Can you work these out from the model? Positions are in its coordinate system, mm. Face numbers are marked on the shaded views. A direction names the side the tool comes from. Give positions to 0.01 mm unless a question says otherwise; leave off trailing zeros. Write each loop counter-clockwise with the first axis right and the second up, starting at its lowest first coordinate (ties: lowest second). Pieces come first, ordered by that corner, then holes.
```python
from build123d import *

# Parameters (mm, degrees)
BOSS_EXTRUDE1_START = -9
BOSS_EXTRUDE1_DEPTH = 82
CHAMFER1_SIZE       = 0.5


with BuildPart() as part:
    # Sketch1 → Boss-Extrude1 (new body)
    with BuildSketch(Plane(origin=(0, 0, 0), x_dir=(0, 0, -1), z_dir=(1, 0, 0)).offset(BOSS_EXTRUDE1_START)):
        Polygon((0, 7.505553499), (-6.5, 3.75277675), (-6.5, -3.75277675), (0, -7.505553499), (6.5, -3.75277675), (6.5, 3.75277675), align=None)
    extrude(amount=BOSS_EXTRUDE1_DEPTH)

    # Sketch2 → Cut-Revolve1 (revolve, cut)
    with BuildSketch(Plane.XY, mode=Mode.PRIVATE) as cut_revolve1_sk:
        Polygon((0, 7.505553499), (-9, 7.505553499), (-9, 4), (-1, 4), (-1, 3.45), (0, 3.45), align=None)
    revolve(cut_revolve1_sk.sketch.rotate(Axis((-20.13204944, 0, 0), (1, 0, 0)), 90), axis=Axis((-20.13204944, 0, 0), (1, 0, 0)), mode=Mode.SUBTRACT)

    # Sketch3 → Cut-Revolve2 (revolve, cut)
    with BuildSketch(Plane.XY, mode=Mode.PRIVATE) as cut_revolve2_sk:
        Polygon((34.8, 7.505553499), (34.8, 4), (35.8, 4), (35.8, 3), (65, 3), (65, 2.5), (73, 2.5), (73, 7.505553499), align=None)
    revolve(cut_revolve2_sk.sketch.rotate(Axis((-14.24617289, 0, 0), (1, 0, 0)), 90), axis=Axis((-14.24617289, 0, 0), (1, 0, 0)), mode=Mode.SUBTRACT)

    # Sketch4 → Cut-Revolve3 (revolve, cut)
    with BuildSketch(Plane.XY, mode=Mode.PRIVATE) as cut_revolve3_sk:
        Polygon((34.8, 7.505553499), (34.075105849, 7.505553499), (34.8, 6.25), align=None)
    revolve(cut_revolve3_sk.sketch.rotate(Axis((-12.936203068, 0, 0), (1, 0, 0)), 90), axis=Axis((-12.936203068, 0, 0), (1, 0, 0)), mode=Mode.SUBTRACT)

    # Chamfer1
    chamfer1_edges = [part.edges().sort_by_distance(p)[0] for p in [
        (-9, 0, -4),
        (73, 0, -2.5),
    ]]
    chamfer(chamfer1_edges, length=CHAMFER1_SIZE)


solid = part.part
```
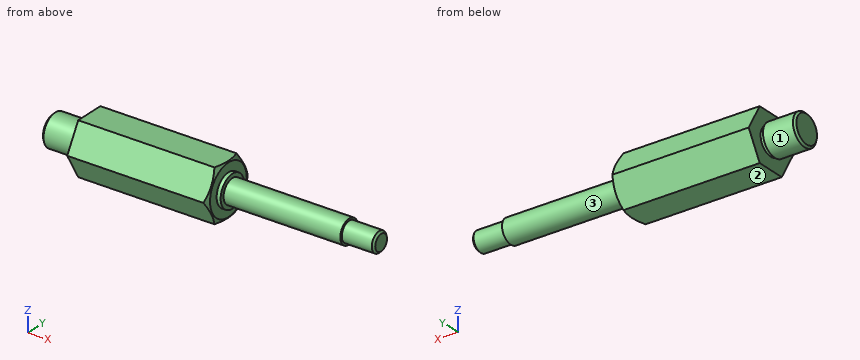
1) Please list where these lines run through material, in increasing order: L1, parallel to X at y = -3.75, z = 4.25; L2, parallel to X at y = 0.5, z = -2.75; L3, parallel to X at y = -0.75, z = 3.75.
Values follow:
L1: x = 0 to 34.8
L2: x = -9 to 65
L3: x = -8.68 to -1, 0 to 35.8
2) For the marked faces 1, 2 and 3, which set-ups out of +Z, -Z, +X, -X, +Y, -Y let a thin tool reach every point of the face, with its end or its side?
Values follow:
face 1: -X
face 2: -Z, +X, -X, +Y, -Y
face 3: +X
3) Suppose I cut it at C-C on x = 67. Write out the boundary of the cut face in (y, z), plus the area to 3 significant figures.
Values follow:
outline: circle Ø5 at (0, 0)
area: 19.6 mm2
4) For pin 1 Ø6 at (y, z) = (3, 1) entering from +X; pin 2 Ø8 at (x, y) = (62, 5.5) entering from +Z; pin 3 Ø4 at (x, y) = (64, -2.5) entering from +Z; pin 4 Ø6 at (x, y) = (60, 3.5) entering from -Z, each with a flat end and sliding along its axis, tell me the tip position at first contact or that it passes through.
Values follow:
pin 1: stops at x = 73
pin 2: stops at z = 2.6
pin 3: stops at z = 2.96
pin 4: stops at z = -2.96
5) Suppose I cut it at D-D on x = 44. Write out the boundary of the cut face in (y, z), plus the area to 3 significant figures.
Values follow:
outline: circle Ø6 at (0, 0)
area: 28.3 mm2
6) Suppose I cut it at A-A on x = 19. Write out the boundary of the cut face in (y, z).
Values follow:
outline: (-7.51, 0) - (-3.75, -6.5) - (3.75, -6.5) - (7.51, 0) - (3.75, 6.5) - (-3.75, 6.5) - close
